Answer from the drawing. Dimensions are ordinates in mm from the lowest x, y and z of the part. Coordinates: 2 decimals unless noted, no trailing zeros. Write each loop counter-clockwise with the first axis right and the second up, starting at its lowest first coordinate (ties: lowest second). Pieces come first, ordered by that corner, then holes. Notation, with made-up numbers: (-15, -6) - (3, -6) arc R29 ccw to (3, 15) - close; hole circle Ø2 at (-25.5, 40.25). An arc over 180 degrees is marked (long way). Return JSON: item names as keys, results as strings.
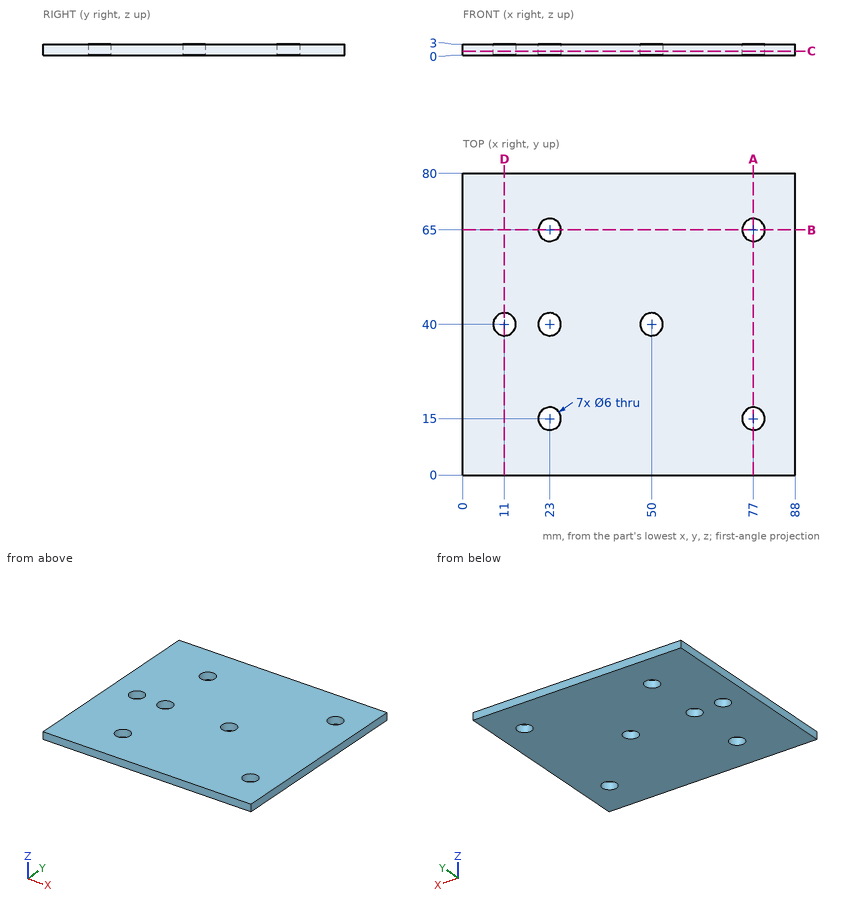
(1) A cutting plane is placed at C-C (z = 1.1). Determine the outline of the cut face in (x, y).
Answer:
{"outline": "(0, 0) - (88, 0) - (88, 80) - (0, 80) - close; hole circle Ø6 at (11, 40); hole circle Ø6 at (23, 15); hole circle Ø6 at (23, 40); hole circle Ø6 at (23, 65); hole circle Ø6 at (50, 40); hole circle Ø6 at (77, 15); hole circle Ø6 at (77, 65)"}
(2) A cutting plane is placed at B-B (y = 65). Determine the outline of the cut face in (x, z), and give its area (3 significant figures).
Answer:
{"outline": "(0, 0) - (20, 0) - (20, 3) - (0, 3) - close; (26, 0) - (74, 0) - (74, 3) - (26, 3) - close; (80, 0) - (88, 0) - (88, 3) - (80, 3) - close", "area": "228 mm²"}
(3) Straight lines are drawn through the part: line 1 (Y direction, x = 77, z = 0.6); line 2 (X direction, y = 40, z = 0.95); line 3 (Y direction, x = 25, z = 1.95). For each, find the intervals that lie inside material, in ascending order. Write a range as from..to.
Answer:
{"line 1": "0..12, 18..62, 68..80", "line 2": "0..8, 14..20, 26..47, 53..88", "line 3": "0..12.76, 17.24..37.76, 42.24..62.76, 67.24..80"}
(4) A cutting plane is placed at A-A (x = 77). Determine the outline of the cut face in (y, z).
Answer:
{"outline": "(0, 0) - (12, 0) - (12, 3) - (0, 3) - close; (18, 0) - (62, 0) - (62, 3) - (18, 3) - close; (68, 0) - (80, 0) - (80, 3) - (68, 3) - close"}
(5) A cutting plane is placed at D-D (x = 11). Determine the outline of the cut face in (y, z), and give its area (3 significant figures).
Answer:
{"outline": "(0, 0) - (37, 0) - (37, 3) - (0, 3) - close; (43, 0) - (80, 0) - (80, 3) - (43, 3) - close", "area": "222 mm²"}
